from build123d import *

# Parameters (mm, degrees)
SKETCH1_W                = 6.35
SKETCH1_H                = 6.35
BOSS_EXTRUDE1_DEPTH      = 152.4
SKETCH2_R                = 1.651
CUT_EXTRUDE1_DEPTH       = 19.05
SKETCH3_R                = 1.651
CUT_EXTRUDE2_DEPTH       = 153.565274965
CHAMFER1_SIZE            = 1.5875
CHAMFER1_OF_MIRROR1_SIZE = 1.5875


with BuildPart() as part:
    # Sketch1 → Boss-Extrude1 (new, symmetric)
    with BuildSketch(Plane(origin=(0, 0, 0), x_dir=(0, 0, -1), z_dir=(1, 0, 0))):
        Rectangle(SKETCH1_W, SKETCH1_H)
    extrude(amount=BOSS_EXTRUDE1_DEPTH, both=True)

    # Sketch2 → Cut-Extrude1 (cut)
    with BuildSketch(Plane(origin=(152.4, 0, 0), x_dir=(0, 0, -1), z_dir=(1, 0, 0))):
        Circle(SKETCH2_R)
    cut_extrude1 = extrude(amount=-CUT_EXTRUDE1_DEPTH, mode=Mode.SUBTRACT)

    # Sketch3 → Cut-Extrude2 (cut, through all)
    with BuildSketch(Plane(origin=(0, -3.175, 0), x_dir=(-1, 0, 0), z_dir=(0, -1, 0))):
        with Locations(Location((-114.3, 0, 0), (0, 0, 90))):
            Circle(SKETCH3_R)
    cut_extrude2 = extrude(amount=-CUT_EXTRUDE2_DEPTH, mode=Mode.SUBTRACT)

    # Chamfer1
    # the kernel refuses this chamfer: 1.5875 mm, written as the material it takes off along each edge
    with BuildSketch(Plane(origin=(114.3, -3.175, 0), x_dir=(0, 0, -1), z_dir=(-1, 0, 0))) as chamfer1_piece_1:
        Polygon((1.651 + CHAMFER1_SIZE, 0), (1.651, -CHAMFER1_SIZE), (1.651, 0), align=None)
    revolve(axis=Axis((114.3, -3.175, 0), (0, -1, 0)), mode=Mode.SUBTRACT)

    # Mirror1: Cut-Extrude1, Cut-Extrude2 across plane
    add(cut_extrude1.mirror(Plane(origin=(0, 0, 0), x_dir=(0, 0, 1), z_dir=(1, 0, 0))), mode=Mode.SUBTRACT)
    add(cut_extrude2.mirror(Plane(origin=(0, 0, 0), x_dir=(0, 0, 1), z_dir=(1, 0, 0))), mode=Mode.SUBTRACT)

    # Chamfer1 of Mirror1
    # the kernel refuses this chamfer: 1.5875 mm, written as the material it takes off along each edge
    with BuildSketch(Plane(origin=(-114.3, -3.175, 0), x_dir=(0, 0, -1), z_dir=(1, 0, 0))) as chamfer1_of_mirror1_piece_1:
        Polygon((1.651 + CHAMFER1_OF_MIRROR1_SIZE, 0), (1.651, CHAMFER1_OF_MIRROR1_SIZE), (1.651, 0), align=None)
    revolve(axis=Axis((-114.3, -3.175, 0), (0, 1, 0)), mode=Mode.SUBTRACT)


solid = part.part
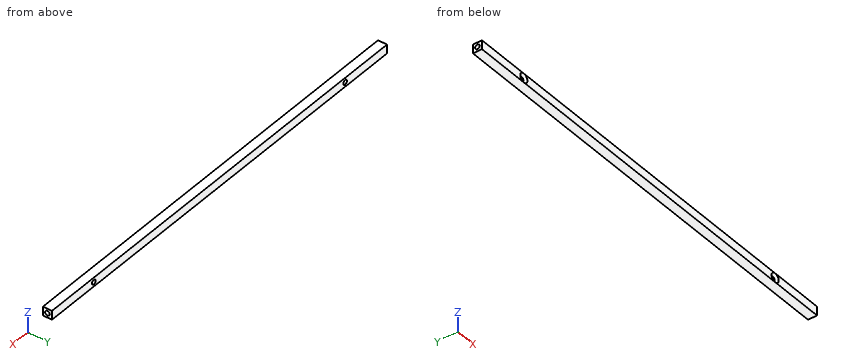
The listing builds one solid part. Answer for the finished solid, in the listing's coordinates (mm). Coordinates: 2 decimals unless noted, no trailing zeros. Write each loop counter-clockwise with the first axis right and the second up, starting at its lowest first coordinate (ties: lowest second). Pieces come first, ordered by that corner, then holes. Notation, with made-up numbers: (36.25, 55) - (78.25, 55) arc R21 cw to (78.25, 92) - close; hole circle Ø1 at (77, 24.25). An arc over 180 degrees is marked (long way). Return JSON: item names as keys, results as strings.
1. The part is cut by section A-A on z = 0. Count the separate pieces of the cut face and the enclosed holes in it, then the cut area to 3 significant figures.
Final values:
{"separate pieces": "3", "enclosed holes": "0", "area": "1,760 mm^2"}
2. The part is cut by section B-B on y = 0. Determine the outline of the cut face in (x, z) (3 decimals), then the cut area to 3 significant figures.
Final values:
{"outline": "(-152.4, -3.175) - (152.4, -3.175) - (152.4, -1.651) - (133.35, -1.651) - (133.35, 1.651) - (152.4, 1.651) - (152.4, 3.175) - (-152.4, 3.175) - (-152.4, 1.651) - (-133.35, 1.651) - (-133.35, -1.651) - (-152.4, -1.651) - close; hole circle Ø3.302 at (-114.3, 0); hole circle Ø3.302 at (114.3, 0)", "area": "1,790 mm^2"}
3. Each of these flat-tipped pins is pushed along its axis until it touches: pin 1 Ø3.5 at (y, z) = (-0.5, 0.5) entering from -X; pin 2 Ø2 at (x, z) = (114.3, 0) entering from +Y; pin 3 Ø3 at (y, z) = (0, 0) entering from +X. Where does it stop, or does it pass through?
Final values:
{"pin 1": "x = -152.4", "pin 2": "through", "pin 3": "x = 133.35"}
4. Consider line 1 along X through (y, z) = (1.05, 0); line 2 along X through (y, z) = (1.5, -1.5); line 3 along Z through (x, y) = (114.3, -0.4) (3 decimals). Determine where each line is inside the solid, lowest interval first.
Final values:
{"line 1": "-133.35 to -115.95, -112.65 to 112.65, 115.95 to 133.35", "line 2": "-152.4 to -114.99, -113.61 to 113.61, 114.99 to 152.4", "line 3": "-3.175 to -1.651, 1.651 to 3.175"}
